Drawing for the job (mm, zero at the part's lowest x, y, z). Give positions to 0.01 mm unless a question says otherwise; leave off trailing zeros. Order: outer loops, then holes, each group sorted by start corner. A loop starts at its lowest first (then second) coordinate and runs counter-clockwise, first axis right, second up. Notation, with made-up numbers: (-1, 2.5) -> (4, 2.5) arc R20 ccw to (4, 30.5) -> close; hole circle Ø11 at (-37.5, -17.5). An arc over 180 degrees is marked (long way). One line per item, written item: value. Start each with the question number.
(1) Saw through at B-B on x = 13. Give the cut face in (y, z).
(2) Probe line 1 (X direction, y = 2.25, z = 11.5); line 2 (Z direction, x = 16, y = 0.2); line 3 (X direction, y = 1.8, z = 7.5) (1 decimal). List the from-to ranges inside material, lowest first.
(3) Saw through at A-A on z = 13. Give the cut face in (x, y), plus the area to 3 significant figures.
(4) Saw through at C-C on y = 1.7. Give the cut face in (x, z).
(5) Pin check, flat tips, straight feed: pin 1 (1 mm diameter, centred on y = 1, z = 20, fed in from -X); pin 2 (1.5 mm diameter, centred on x = 9, y = 1.5, fed in from +Z); pin 3 (1 mm diameter, centred on x = 14, y = 1.5, fed in from -Z); pin 4 (3 mm diameter, centred on x = 4, z = 21, fed in from +Y). Stop position of each tip, or through.
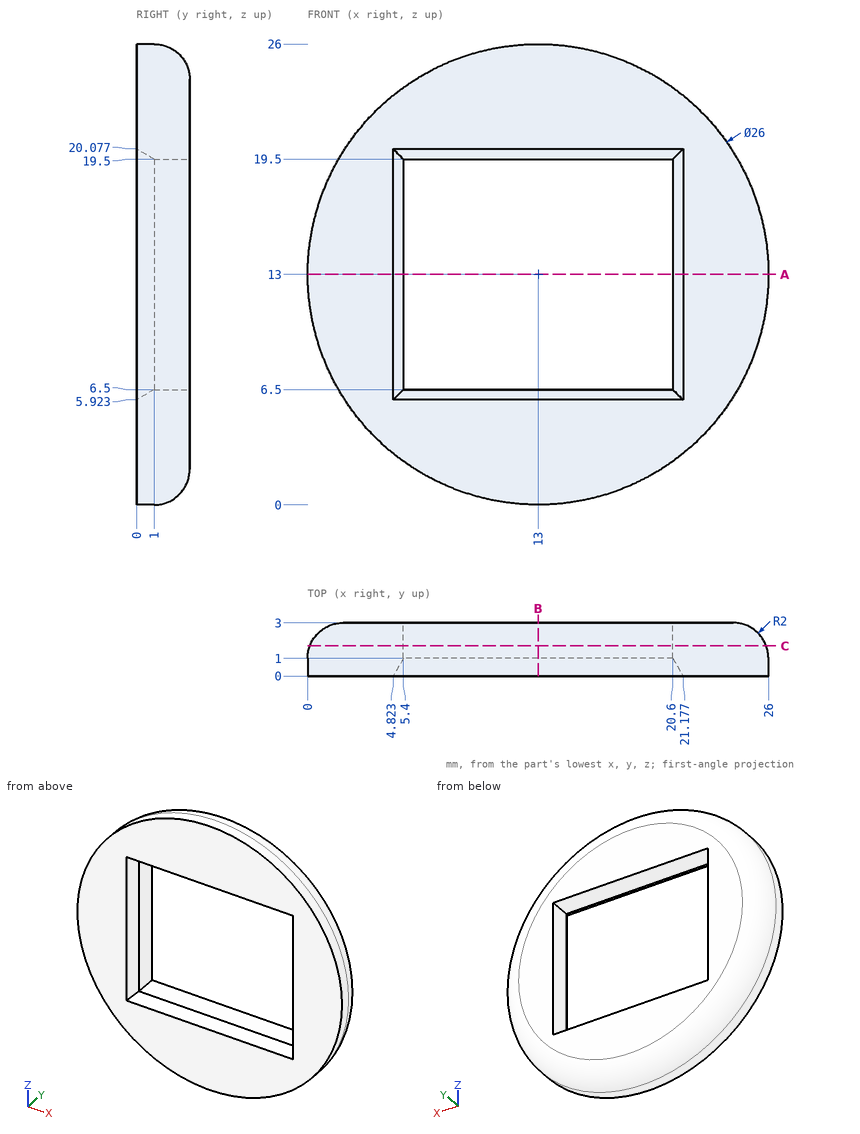
Results below:
1. outline: (0, 0) -> (1, 0) arc R2 ccw to (3, 2) -> (3, 6.5) -> (1, 6.5) -> (0, 5.92) -> close; (0, 20.08) -> (1, 19.5) -> (3, 19.5) -> (3, 24) arc R2 ccw to (1, 26) -> (0, 26) -> close
2. line 1: x = 0.53 to 5.4, 20.6 to 25.47
2. line 2: z = 0.35 to 6.04, 19.96 to 25.65
2. line 3: x = 1.4 to 5.4, 20.6 to 24.6
3. outline: (0, 0) -> (4.82, 0) -> (5.4, 1) -> (5.4, 3) -> (2, 3) arc R2 ccw to (0, 1) -> close; (20.6, 1) -> (21.18, 0) -> (26, 0) -> (26, 1) arc R2 ccw to (24, 3) -> (20.6, 3) -> close
3. area: 30.1 mm²
4. outline: circle Ø25.75 at (13, 13); hole (5.4, 6.5) -> (20.6, 6.5) -> (20.6, 19.5) -> (5.4, 19.5) -> close
5. pin 1: stops at x = 1.74
5. pin 2: stops at z = 25.56
5. pin 3: stops at z = 0.02
5. pin 4: stops at y = 3
